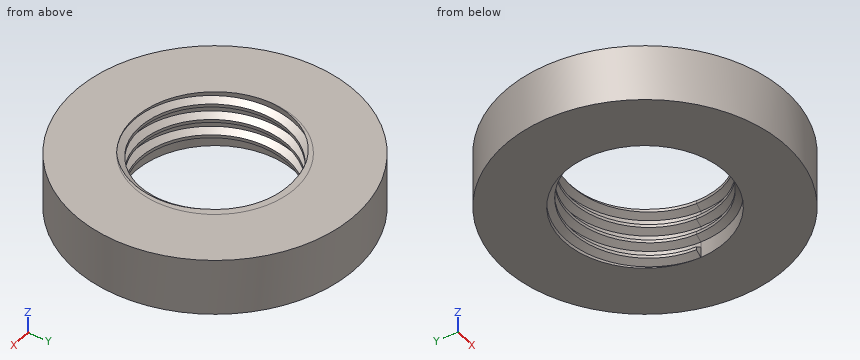
```python
from build123d import *

# Parameters (mm, degrees)
SKETCH1_R           = 17.5
SKETCH1_R_2         = 10
BOSS_EXTRUDE1_DEPTH = 7
THREAD1_PITCH       = 2
SKETCH4_W           = 35
SKETCH4_H           = 2.231433202
CUT_EXTRUDE1_DEPTH  = 28.5


with BuildPart() as part:
    # Sketch1 → Boss-Extrude1 (new body)
    with BuildSketch(Plane.XY):
        Circle(SKETCH1_R)
        Circle(SKETCH1_R_2, mode=Mode.SUBTRACT)
    extrude(amount=BOSS_EXTRUDE1_DEPTH)

    # Thread1: the profile of Thread Profile1 profile screwed along a right-hand helix of 3.5 turns, 10 arcs to a turn; built about Z, then put on its axis
    thread1_z = Axis((0, 0, 0), (0, 0, 1))
    thread1_corners = [(10.0003, 0, -0.000173205), (10.0003, 0, 1.312673201), (9.188101187, 0, 0.843749998), (9.188101187, 0, 0.468749998)]
    with BuildLine(mode=Mode.PRIVATE) as thread1_profile:
        Line(thread1_corners[0], thread1_corners[1])
        Line(thread1_corners[1], thread1_corners[2])
        Line(thread1_corners[2], thread1_corners[3])
        Line(thread1_corners[3], thread1_corners[0])
    thread1_cap = Face(thread1_profile.wire())
    thread1_turn_angles = [0, 18, 36, 54, 72, 90, 108, 126, 144, 162, 180, 198, 216, 234, 252, 270, 288, 306, 324, 342, 360]
    thread1_turn_weights = [1, 0.9510565162951535, 1, 0.9510565162951535, 1, 0.9510565162951535, 1, 0.9510565162951535, 1, 0.9510565162951535, 1, 0.9510565162951535, 1, 0.9510565162951535, 1, 0.9510565162951535, 1, 0.9510565162951535, 1, 0.9510565162951535, 1]
    thread1_turn_rails = [Edge.make_bspline([Vector(p[0], p[1], 0).rotate(thread1_z, thread1_turn_angles[k]) / thread1_turn_weights[k] + Vector(0, 0, p[2] + THREAD1_PITCH * thread1_turn_angles[k] / 360) for k in range(21)], [0, 0, 0, 1, 1, 2, 2, 3, 3, 4, 4, 5, 5, 6, 6, 7, 7, 8, 8, 9, 9, 10, 10, 10], 2, thread1_turn_weights) for p in thread1_corners]
    thread1_turn_sides = [Face.make_surface_from_curves(thread1_turn_rails[p[0]], thread1_turn_rails[p[1]]) for p in [(0, 1), (1, 2), (2, 3), (3, 0)]]
    thread1_last_angles = [1080, 1098, 1116, 1134, 1152, 1170, 1188, 1206, 1224, 1242, 1260]
    thread1_last_weights = [1, 0.9510565162951535, 1, 0.9510565162951535, 1, 0.9510565162951535, 1, 0.9510565162951535, 1, 0.9510565162951535, 1]
    thread1_last_rails = [Edge.make_bspline([Vector(p[0], p[1], 0).rotate(thread1_z, thread1_last_angles[k]) / thread1_last_weights[k] + Vector(0, 0, p[2] + THREAD1_PITCH * thread1_last_angles[k] / 360) for k in range(11)], [0, 0, 0, 1, 1, 2, 2, 3, 3, 4, 4, 5, 5, 5], 2, thread1_last_weights) for p in thread1_corners]
    thread1_last_sides = [Face.make_surface_from_curves(thread1_last_rails[p[0]], thread1_last_rails[p[1]]) for p in [(0, 1), (1, 2), (2, 3), (3, 0)]]
    thread1 = Plane(origin=(0, 0, 0), x_dir=(1, 0, 0), z_dir=(0, 0, 1)) * Solid(Shell([*[p.moved(Location((0, 0, THREAD1_PITCH * i))) for i in range(3) for p in thread1_turn_sides], *thread1_last_sides, thread1_cap, thread1_cap.rotate(thread1_z, 1260).moved(Location((0, 0, THREAD1_PITCH * 1260 / 360)))]))
    add(thread1)

    # Sketch4 → Cut-Extrude1 (cut, symmetric)
    with BuildSketch(Plane(origin=(0, 0, 0), x_dir=(1, 0, 0), z_dir=(0, 1, 0))):
        with Locations((0, -8.115716601)):
            Rectangle(SKETCH4_W, SKETCH4_H)
    extrude(amount=CUT_EXTRUDE1_DEPTH, both=True, mode=Mode.SUBTRACT)


solid = part.part
```
Here's how the part is built. I have some questions about the finished solid (model axes, mm). Coordinates: 2 decimals unless noted, no trailing zeros. Order: outer loops, then holes, each group sorted by start corner. A loop starts at its lowest first (then second) coordinate and runs counter-clockwise, first axis right, second up. Notation, with made-up numbers: (-23.75, 68) - (30.25, 68) arc R17 cw to (30.25, 85) - close; hole circle Ø2 at (22.25, 12). An arc over 180 degrees is marked (long way). One line per question, with ' | ' between items.
(1) Suppose I cut it at B-B on y = -12. List the corners of the cut face in (x, z) for me.
Report:
outline: (-12.74, 0) - (12.74, 0) - (12.74, 7) - (-12.74, 7) - close
(2) Suppose I cut it at A-A on x = -11. List the corners of the cut face in (y, z) for me, and give its area (3 significant figures).
Report:
outline: (-13.61, 0) - (13.61, 0) - (13.61, 7) - (-13.61, 7) - close | area: 191 mm2
(3) If I drill on L1, parallel to Y at x = 0, z = 1.3; L2, parallel to X at y = 0, z = 5.7; L3, parallel to X at y = 0, z = 1.9, over which ranges is the centre line in solid material (lowest first)?
Report:
L1: y = -17.5 to -10, 9.19 to 17.5 | L2: x = -17.5 to -9.19, 10 to 17.5 | L3: x = -17.5 to -9.29, 10 to 17.5
(4) Will these pins go through, and if not, where does the flat tip stop? pin 1 (1 mm diameter, centred on y = 11.5, z = 1.5, fed in from -X); pin 2 (18 mm diameter, centred on x = 0, y = 0, fed in from +Z); pin 3 (1.5 mm diameter, centred on y = 1.5, z = 2, fed in from +X); pin 4 (1 mm diameter, centred on y = 9, z = 2.5, fed in from -X).
Report:
pin 1: stops at x = -13.61 | pin 2: passes through | pin 3: stops at x = 17.48 | pin 4: stops at x = -15.3
